Input: part model. Units: mm. Frame: model coordinates. A direction names the side the tool comes from. Coordinates: 2 decimals unless noted, no trailing zeros. Order: outer loops, then holes, each group sorted by start corner. A loop starts at its lowest first (then second) coordinate and runs counter-clockwise, first axis right, second up.
from build123d import *

# Parameters (mm, degrees)
HOLE_WIZARD_M3_1_D           = 2.5
CHAMFER_1_SIZE               = 1
CHAMFER_2_SIZE               = 0.5
CHAMFER_2_SIZE2              = 0.288675135
CHAMFER_2_PART_2_SIZE        = 0.5
CHAMFER_2_PART_2_SIZE2       = 0.288675135
CHAMFER_2_PART_3_SIZE        = 0.5
CHAMFER_2_PART_3_SIZE2       = 0.288675135
HOLE_WIZARD_M3_2_D           = 2.5
HOLE_WIZARD_M3_2_DEPTH       = 6
HOLE_WIZARD_M3_2_CSINK_D     = 3.5
HOLE_WIZARD_M3_2_CSINK_ANGLE = 90
HOLE_WIZARD_M3_2_TIP         = 0.751075774


with BuildPart() as part:
    # 草图2 → 旋转1 (revolve)
    with BuildSketch(Plane.XY):
        Polygon((3.25, 0), (8.5, 0), (8.5, 5), (9, 5), (9, 6), (3.25, 6), (3.25, 49.5), (9, 49.5), (9, 54.5), (1.25, 54.5), (1.25, -11.5), (2.25, -11.5), (2.25, -6.5), (3.25, -6.5), align=None)
    revolve(axis=Axis((0, 60, 0), (0, -1, 0)))

    # M3 螺纹孔1 (through all)
    with Locations(Plane(origin=(0, 54.5, 0), x_dir=(1, 0, 0), z_dir=(0, 1, 0))):
        with Locations((-5.196152423, -3), (0, 6), (5.196152423, -3)):
            Hole(HOLE_WIZARD_M3_1_D / 2)

    # 倒角1
    chamfer_1_edges = [part.edges().sort_by_distance(p)[0] for p in [
        (-3.25, 6, 0),
        (-3.25, 49.5, 0),
    ]]
    chamfer(chamfer_1_edges, length=CHAMFER_1_SIZE)

    # 倒角2
    chamfer_2_edges = [part.edges().sort_by_distance(p)[0] for p in [
        (-9, 49.5, 0),
    ]]
    chamfer_2_side = [part.faces().sort_by_distance(p)[0] for p in [
        (-4.504558441, 49.5, 0),
    ]]
    chamfer(chamfer_2_edges, length=CHAMFER_2_SIZE, length2=CHAMFER_2_SIZE2, reference=chamfer_2_side[0])

    # 倒角2 part 2
    chamfer_2_part_2_edges = [part.edges().sort_by_distance(p)[0] for p in [
        (-9, 54.5, 0),
    ]]
    chamfer_2_part_2_side = [part.faces().sort_by_distance(p)[0] for p in [
        (-9, 52, 0),
    ]]
    chamfer(chamfer_2_part_2_edges, length=CHAMFER_2_PART_2_SIZE, length2=CHAMFER_2_PART_2_SIZE2, reference=chamfer_2_part_2_side[0])

    # 倒角2 part 3
    chamfer_2_part_3_edges = [part.edges().sort_by_distance(p)[0] for p in [
        (-2.25, -11.5, 0),
    ]]
    chamfer_2_part_3_side = [part.faces().sort_by_distance(p)[0] for p in [
        (-1.31363961, -11.5, 0),
    ]]
    chamfer(chamfer_2_part_3_edges, length=CHAMFER_2_PART_3_SIZE, length2=CHAMFER_2_PART_3_SIZE2, reference=chamfer_2_part_3_side[0])

    # M3 螺纹孔2
    with Locations(Plane(origin=(0, 54.5, 0), x_dir=(1, 0, 0), z_dir=(0, 1, 0))):
        with Locations((0, 0)):
            CounterSinkHole(HOLE_WIZARD_M3_2_D / 2, HOLE_WIZARD_M3_2_CSINK_D / 2, depth=HOLE_WIZARD_M3_2_DEPTH, counter_sink_angle=HOLE_WIZARD_M3_2_CSINK_ANGLE)
            with Locations((0, 0, -(HOLE_WIZARD_M3_2_DEPTH + HOLE_WIZARD_M3_2_TIP / 2))):  # 118° drill point
                Cone(0, HOLE_WIZARD_M3_2_D / 2, HOLE_WIZARD_M3_2_TIP, mode=Mode.SUBTRACT)


solid = part.part
Item 1: Draft query along Y for faces 1 (the face through (-1.172, 51.924, 8.923)), 2 (the face through (0, 54.5, -2)), 3 (the face through (4, 49.5, -2)). Return one class per face: pulls with the +Y half, pulls with the -Y half, needs draft (parallel to the pull), parting line crosses it, or undercut.
Response values:
face 1: needs draft
face 2: pulls with the +Y half
face 3: undercut
Item 2: Cut plane A-A on x = 0. Count the separate pieces of the cut face and the enclosed holes in it, then the cut area to 3 significant figures.
Response values:
separate pieces: 4
enclosed holes: 0
area: 349 mm2
Item 3: Ray query, probe 1 along Z at (x, y) = (0, 3.45); probe 2 along Z at (x, y) = (0, 29.5); probe 3 along Z at (x, y) = (0, 52.4). Return the intervals inside material, ascending.
Response values:
probe 1: z = -8.5 to -7.25, -4.75 to -1.25, 1.25 to 8.5
probe 2: z = -3.25 to -1.25, 1.25 to 3.25
probe 3: z = -9 to -7.25, -4.75 to -1.25, 1.25 to 9
Item 4: Pin query (flat end, axial travel): pin 1 Ø8 at (x, z) = (3.5, 4) entering from -Y; pin 2 Ø3 at (x, z) = (5.2, 3) entering from -Y; pin 3 Ø3 at (x, y) = (3.5, 16.5) entering from -Z; pin 4 Ø8 at (y, z) = (34, -3) entering from +X. Return the tip coordinate at first contact, or that it passes through.
Response values:
pin 1: stops at y = -11.5
pin 2: stops at y = 0
pin 3: stops at z = -2.56
pin 4: stops at x = 3.25
Item 5: Access query for faces 4 (the face through (-4.27, 51.96, 2.16)), 5 (the face through (-2.579, 28.04, -1.978)), 6 (the face through (-8, 5, -3.3)). Directions: +Z, -Z, +X, -X, +Y, -Y. A direction counts if a zero-diameter tool reaches every point of the face in a straight line with its end or side. Return the directions, or none.
Response values:
face 4: +Y, -Y
face 5: none
face 6: -Y
Item 6: Cut plane B-B on y = 33. Return loops of the section in (x, z), then the cut area to 3 significant figures.
Response values:
outline: circle Ø6.5 at (0, 0); hole circle Ø2.5 at (0, 0)
area: 28.3 mm2
